Design review of the part built by this model. Coordinates are the model's own, in mm. A direction names the side the tool comes from. Give positions to 0.01 mm unless a question says otherwise; leave off trailing zeros. Write each loop counter-clockwise with the first axis right and the second up, starting at its lowest first coordinate (ties: lowest second). Pieces come first, ordered by that corner, then holes. Notation, with made-up numbers: (75, 59) -> (100, 59) arc R26 cw to (100, 89) -> close; hole circle Ø7 at (-35.75, -38.5). An arc over 180 degrees is marked (long way). Answer as a JSON object with one key per item and string values.
```python
from build123d import *

# Parameters (mm, degrees)
BOSS_EXTRUDE1_DEPTH = 7.62
SKETCH4_3_R         = 1.5
BOSS_EXTRUDE2_DEPTH = 2.54
SKETCH5_W           = 60.579
SKETCH5_H           = 7.62
BOSS_EXTRUDE3_DEPTH = 2.54
FILLET1_R           = 15.24
FILLET2_R           = 5.08
FILLET3_R           = 2.54


with BuildPart() as part:
    # Sketch4 → Boss-Extrude1 (new body)
    with BuildSketch(Plane.XY):
        with BuildLine():
            Line((34.731702618, -14.493095403), (-3.368297382, -14.493095403))
            Line((-3.368297382, -14.493095403), (-3.368297382, 5.191904597))
            ThreePointArc((-3.368297382, 5.191904597), (-0.020527891, 13.274135106), (8.061702618, 16.621904597))
            Line((8.061702618, 16.621904597), (34.731702618, 16.621904597))
            Line((34.731702618, 16.621904597), (34.731702618, 20.050904597))
            Line((34.731702618, 20.050904597), (8.061702618, 20.050904597))
            ThreePointArc((8.061702618, 20.050904597), (-2.445197043, 15.698804259), (-6.797297382, 5.191904597))
            Line((-6.797297382, 5.191904597), (-6.797297382, -5.10519069))
            Line((-6.797297382, -5.10519069), (-25.847297382, -21.160595403))
            Line((-25.847297382, -21.160595403), (34.731702618, -21.160595403))
            Line((34.731702618, -21.160595403), (34.731702618, -14.493095403))
        make_face()
    extrude(amount=-BOSS_EXTRUDE1_DEPTH)

    # Sketch4_3 → Boss-Extrude2 (add)
    with BuildSketch(Plane.XY):
        with BuildLine():
            Line((-3.368297382, -11.064095403), (-3.368297382, -14.493095403))
            Line((-3.368297382, -14.493095403), (34.731702618, -14.493095403))
            Line((34.731702618, -14.493095403), (34.731702618, 16.621904597))
            Line((34.731702618, 16.621904597), (8.061702618, 16.621904597))
            ThreePointArc((8.061702618, 16.621904597), (-0.020527891, 13.274135106), (-3.368297382, 5.191904597))
            Line((-3.368297382, 5.191904597), (-3.368297382, -8.326281589))
            Line((-3.368297382, -8.326281589), (-3.368297382, -11.064095403))
        make_face()
        with Locations((5.973177543, -3.081984913)):
            Circle(SKETCH4_3_R, mode=Mode.SUBTRACT)
        with Locations((18.742087817, -4.794749031)):
            Circle(SKETCH4_3_R, mode=Mode.SUBTRACT)
        with Locations((5.712659725, 8.949609908)):
            Circle(SKETCH4_3_R, mode=Mode.SUBTRACT)
        with Locations((17.97317096, 7.733253911)):
            Circle(SKETCH4_3_R, mode=Mode.SUBTRACT)
    extrude(amount=-BOSS_EXTRUDE2_DEPTH)

    # Sketch5 → Boss-Extrude3 (add)
    with BuildSketch(Plane.XZ.offset(21.160595403)):
        with Locations((4.442202618, -3.81)):
            Rectangle(SKETCH5_W, SKETCH5_H)
    extrude(amount=BOSS_EXTRUDE3_DEPTH)

    # Fillet1
    fillet1_edges = [part.edges().sort_by_distance(p)[0] for p in [
        (34.731702618, 20.050904597, -3.81),
        (34.731702618, -23.700595403, -3.81),
    ]]
    fillet(fillet1_edges, radius=FILLET1_R)

    # Fillet2
    fillet2_edges = [part.edges().sort_by_distance(p)[0] for p in [
        (-25.847297382, -21.160595403, -3.81),
    ]]
    fillet(fillet2_edges, radius=FILLET2_R)

    # Fillet3
    fillet3_edges = [part.edges().sort_by_distance(p)[0] for p in [
        (-6.797297382, -5.10519069, -3.81),
    ]]
    fillet(fillet3_edges, radius=FILLET3_R)


solid = part.part
```
(1) For faces 1 (the flat face through (15, 1, -2.54)), 2 (the flat face through (34.732, -2, -1)), list the 3-axis set-ups (+Z, -Z, +X, -X, +Y, -Y) from which the entire face can be reached by the end or side of a thin tool; tool diameter is ignored.
Here are the results:
{"face 1": "-Z, +X", "face 2": "+Z, -Z, +X, +Y, -Y"}
(2) For line 1 along X through (y, z) = (8, -1.25); line 2 along X through (y, z) = (-3, -1.5); line 3 along Z through (x, y) = (18.5, 0.5), list the stretches that pass through material, from the lowest coordinate up.
Here are the results:
{"line 1": "x = -6.53 to 4.55, 6.87 to 16.5, 19.45 to 34.39", "line 2": "x = -6.8 to 4.48, 7.47 to 34.73", "line 3": "z = -2.54 to 0"}
(3) We need section D-D, the plane y = 2.5. State the section outline as (x, z) points, then the cut area to 3 significant figures.
Here are the results:
{"outline": "(-6.8, -7.62) -> (-3.37, -7.62) -> (-3.37, -2.54) -> (34.73, -2.54) -> (34.73, 0) -> (-6.8, 0) -> close", "area": "123 mm²"}
(4) We need section C-C, the plane x = -2.5. State the section outline as (y, z) points, then the cut area to 3 significant figures.
Here are the results:
{"outline": "(-23.7, -7.62) -> (-14.49, -7.62) -> (-14.49, -2.54) -> (9.56, -2.54) -> (9.56, -7.62) -> (15.64, -7.62) -> (15.64, 0) -> (-23.7, 0) -> close", "area": "178 mm²"}
(5) We need section B-B, the plane z = -1.5. State the section outline as (x, y) points.
Here are the results:
{"outline": "(-25.85, -23.7) -> (19.49, -23.7) arc R15.24 ccw to (34.73, -8.46) -> (34.73, 4.81) arc R15.24 ccw to (19.49, 20.05) -> (8.06, 20.05) arc R14.86 ccw to (-6.8, 5.19) -> (-6.8, -3.92) arc R2.54 cw to (-7.7, -5.87) -> (-24.04, -19.64) arc R5.08 ccw to (-25.85, -23.52) -> close; hole circle Ø3 at (5.71, 8.95); hole circle Ø3 at (5.97, -3.08); hole circle Ø3 at (17.97, 7.73); hole circle Ø3 at (18.74, -4.79)"}
(6) The part is to be moulded in two halves that separate along X. For faces 3 (the cylindrical face through (20.17, -4.34, -1.25)), 4 (the cylindrical face through (4.868, -2.068, -1.252)), 5 (the cylindrical face through (-0.109, 13.185, -5.044)), 6 (the flat face through (15, -14.493, -5)), say which applies: +X half, -X half, draft (parallel to the pull), parting line (faces both ways), or undercut.
Here are the results:
{"face 3": "undercut", "face 4": "undercut", "face 5": "+X half", "face 6": "draft"}
(7) We need section A-A, the plane z = -5.25. State the section outline as (x, y) points, then the cut area to 3 significant figures.
Here are the results:
{"outline": "(-25.85, -23.7) -> (19.49, -23.7) arc R15.24 ccw to (33.49, -14.49) -> (-3.37, -14.49) -> (-3.37, 5.19) arc R11.43 cw to (8.06, 16.62) -> (29.12, 16.62) arc R15.24 ccw to (19.49, 20.05) -> (8.06, 20.05) arc R14.86 ccw to (-6.8, 5.19) -> (-6.8, -3.92) arc R2.54 cw to (-7.7, -5.87) -> (-24.04, -19.64) arc R5.08 ccw to (-25.85, -23.52) -> close", "area": "736 mm²"}
(8) Clearance check with flat-ended pins moving along their axes: pin 1 (1.8 mm diameter, centred on x = 17.97, y = 7.73, fed in from -Z); pin 2 (3.5 mm diameter, centred on x = 18.74, y = -4.79, fed in from -Z); pin 3 (3 mm diameter, centred on y = -10, z = -6, fed in from -X); pin 4 (2.5 mm diameter, centred on y = -4, z = -6.5, fed in from +X). State where each tip first meets the part, or that it passes through.
Here are the results:
{"pin 1": "passes through", "pin 2": "stops at z = -2.54", "pin 3": "stops at x = -14.38", "pin 4": "stops at x = -3.37"}
